Source: CAD feature listing. Evaluate the final solid. Frame: model axes, mm. Face numbers are marked on the shaded views. A direction names the side the tool comes from. Coordinates: 2 decimals unless noted, no trailing zeros. Order: outer loops, then holes, each group sorted by start corner. A loop starts at its lowest first (then second) coordinate and runs counter-clockwise, first axis right, second up.
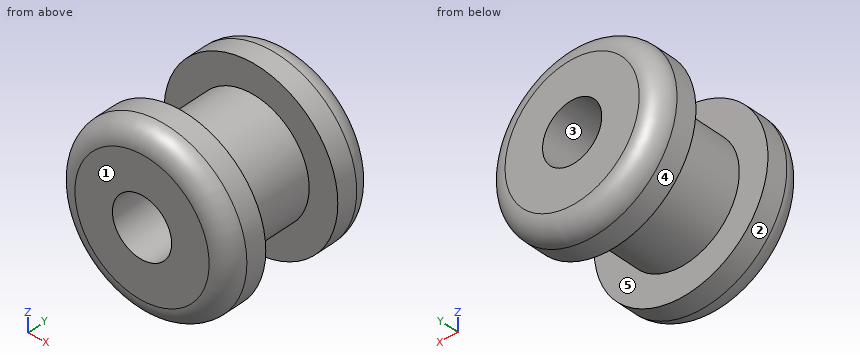
Autodesk Inventor part; units mm, degrees
ref_plane "YZ Plane" through (0, 0, 0) normal (1, 0, 0) x (0, 1, 0)
ref_plane "XZ Plane" through (0, 0, 0) normal (0, 1, 0) x (-1, 0, 0)
ref_plane "XY Plane" through (0, 0, 0) normal (0, 0, 1) x (1, 0, 0)
sketch "Sketch1" plane through (0, 0, 0) normal (0, 0, 1) x (1, 0, 0)
  line L0 (1.5, 0) -> (1.5, 4.05)
  line L1 (1.5, 4.05) -> (4.4, 4.05)
  line L2 (4.4, 4.05) -> (4.4, 2)
  line L3 (4.4, 2) -> (2.95, 2)
  line L4 (2.95, 2) -> (2.95, 0)
  line L5 (0, 0) -> (18.7234, 0) construction
  line L6 (0, 16.7698) -> (0, -15.2532)
  line L7 (1.5, 0) -> (1.5, -4.05)
  line L8 (1.5, -4.05) -> (4.4, -4.05)
  line L9 (4.4, -4.05) -> (4.4, -2)
  line L10 (4.4, -2) -> (2.95, -2)
  line L11 (2.95, -2) -> (2.95, 0)
  dimension "d1" = 0
  dimension "d3" = 3
  dimension "d4" = 5.9
  dimension "d5" = 8.8
  dimension "d6" = 8.1
  dimension "d7" = 4
revolve "Revolution1" add sketch "Sketch1" angle 360 about axis through (0, 16.7698, 0) along (0, -1, 0)
fillet "Fillet1" radius 1 1 edges at (-4.4, 4.05, 0)
fillet "Fillet2" radius 1 1 edges at (-4.4, -4.05, 0)
properties part number "Grommet"
1. Section query D-D on y = -2.25. Return loops of the section in (x, z), plus the area to 3 significant figures.
Findings:
outline: circle Ø8.8 at (0, 0); hole circle Ø3 at (0, 0)
area: 53.8 mm2
2. Section query C-C on y = 0. Return loops of the section in (x, z).
Findings:
outline: circle Ø5.9 at (0, 0); hole circle Ø3 at (0, 0)
3. Ray query, line 1 (Z direction, x = 0, y = -1); line 2 (Z direction, x = 0, y = -2.5); line 3 (Y direction, x = 2.75, z = 1.5). Return the intervals inside material, ascending.
Findings:
line 1: z = -2.95 to -1.5, 1.5 to 2.95
line 2: z = -4.4 to -1.5, 1.5 to 4.4
line 3: y = -4.05 to -2, 2 to 4.05
4. Draft query along Z for the marked faces 1, 2 and 3. Return one class per face: released by +Z, released by -Z, zero draft, split by the parting line, or undercut.
Findings:
face 1: zero draft
face 2: split by the parting line
face 3: undercut
5. Section query A-A on x = 0. Return loops of the section in (y, z).
Findings:
outline: (-4.05, -3.4) arc R1 ccw to (-3.05, -4.4) - (-2, -4.4) - (-2, -2.95) - (2, -2.95) - (2, -4.4) - (3.05, -4.4) arc R1 ccw to (4.05, -3.4) - (4.05, -1.5) - (-4.05, -1.5) - close; (-4.05, 1.5) - (4.05, 1.5) - (4.05, 3.4) arc R1 ccw to (3.05, 4.4) - (2, 4.4) - (2, 2.95) - (-2, 2.95) - (-2, 4.4) - (-3.05, 4.4) arc R1 ccw to (-4.05, 3.4) - close
6. Access query for the marked faces 4 and 5. Directions: +Z, -Z, +X, -X, +Y, -Y. A direction counts if a zero-diameter tool reaches every point of the face in a straight line with its end or side. Return the directions, or none.
Findings:
face 4: +Y, -Y
face 5: none
7. Pin query (flat end, axial travel): P1, Ø3, axis at x = -0.5, z = -1, coming from the +Y side; P2, Ø1, axis at x = 3, y = 0, coming from the +Z side. Return the tip coordinate at first contact, or that it passes through.
Findings:
P1: stops at y = 4.05
P2: stops at z = 1.57
8. Section query B-B on z = 0. Return loops of the section in (x, y).
Findings:
outline: (-4.4, -3.05) arc R1 ccw to (-3.4, -4.05) - (-1.5, -4.05) - (-1.5, 4.05) - (-3.4, 4.05) arc R1 ccw to (-4.4, 3.05) - (-4.4, 2) - (-2.95, 2) - (-2.95, -2) - (-4.4, -2) - close; (1.5, -4.05) - (3.4, -4.05) arc R1 ccw to (4.4, -3.05) - (4.4, -2) - (2.95, -2) - (2.95, 2) - (4.4, 2) - (4.4, 3.05) arc R1 ccw to (3.4, 4.05) - (1.5, 4.05) - close
